Check sheet for the modelled part. Datum: model origin and axes. Units: mm. Give positions to 0.01 mm unless a question says otherwise; leave off trailing zeros. Write each loop counter-clockwise with the first axis right and the second up, starting at its lowest first coordinate (ties: lowest second). Pieces come first, ordered by that corner, then holes. Notation, with made-up numbers: (-16.5, 68.25) -> (20.5, 68.25) arc R27 cw to (20.5, 104.25) -> close; hole circle Ø8 at (-23, 48). An arc over 180 degrees is marked (long way). Use a Markdown table: item, result. Add a question column.
1. Cross-section at A-A (x = 96). Enter the section's corners in (y, z) (3 decimals).
2. Gauge pin test, flat ends, axial feed: P1, Ø10, axis at x = 73, y = 5.5, coming from the -Z side; P2, Ø4, axis at x = 53.5, z = -3.5, coming from the +Y side; P3, Ø4, axis at x = 69, y = -4.5, coming from the +Z side. Record the tip position at first contact, or that the pin passes through.
3. Scan lines: probe 1 along Y at (x, z) = (25, 6); probe 2 along Y at (x, z) = (99.5, 5.75); probe 3 along Z at (x, y) = (114, -4.75). Record each from-to range of solid material in increasing order. Write a range as [from, to].
from build123d import *

# Parameters (mm, degrees)
SKETCH1_W           = 120.675
SKETCH1_H           = 1.5875
CUT_EXTRUDE2_START  = 19.25
SKETCH4_R           = 12.7
CUT_EXTRUDE2_DEPTH  = 22.225
SKETCH6_R           = 7.9375
BOSS_EXTRUDE1_DEPTH = 101.6
SKETCH7_R           = 23.308025585
CUT_EXTRUDE3_DEPTH  = 19.075


with BuildPart() as part:
    # Sketch1 → Revolve1 (revolve)
    with BuildSketch(Plane(origin=(0, 0, 0), x_dir=(1, 0, 0), z_dir=(0, 1, 0))):
        with Locations((79.5875, 8.73125)):
            Rectangle(SKETCH1_W, SKETCH1_H)
    revolve(axis=Axis((157.324, 0, 0), (-1, 0, 0)))

    # Sketch4 → Cut-Extrude2 (cut)
    with BuildSketch(Plane(origin=(0, 0, 0), x_dir=(0, 0, -1), z_dir=(1, 0, 0)).offset(CUT_EXTRUDE2_START)):
        Circle(SKETCH4_R)
        Polygon((-9.235721046, 0.808020891), (-8.681700155, 0.254), (-8.681700155, -0.254), (-9.235721046, -0.808020891), (-8.593912259, -1.257420242), (-8.505698985, -1.75770258), (-8.955098336, -2.399511367), (-8.245002688, -2.730634406), (-8.071256455, -3.207998257), (-8.402379494, -3.918093905), (-7.645572882, -4.120879625), (-7.391572882, -4.56082053), (-7.594358603, -5.317627141), (-6.813836213, -5.385914002), (-6.487300108, -5.775064579), (-6.555586968, -6.555586968), (-5.775064579, -6.487300108), (-5.385914002, -6.813836213), (-5.317627141, -7.594358603), (-4.56082053, -7.391572882), (-4.120879625, -7.645572882), (-3.918093905, -8.402379494), (-3.207998257, -8.071256455), (-2.730634406, -8.245002688), (-2.399511367, -8.955098336), (-1.75770258, -8.505698985), (-1.257420242, -8.593912259), (-0.808020891, -9.235721046), (-0.254, -8.681700155), (0.254, -8.681700155), (0.808020891, -9.235721046), (1.257420242, -8.593912259), (1.75770258, -8.505698985), (2.399511367, -8.955098336), (2.730634406, -8.245002688), (3.207998257, -8.071256455), (3.918093905, -8.402379494), (4.120879625, -7.645572882), (4.56082053, -7.391572882), (5.317627141, -7.594358603), (5.385914002, -6.813836213), (5.775064579, -6.487300108), (6.555586968, -6.555586968), (6.487300108, -5.775064579), (6.813836213, -5.385914002), (7.594358603, -5.317627141), (7.391572882, -4.56082053), (7.645572882, -4.120879625), (8.402379494, -3.918093905), (8.071256455, -3.207998257), (8.245002688, -2.730634406), (8.955098336, -2.399511367), (8.505698985, -1.75770258), (8.593912259, -1.257420242), (9.235721046, -0.808020891), (8.681700155, -0.254), (8.681700155, 0.254), (9.235721046, 0.808020891), (8.593912259, 1.257420242), (8.505698985, 1.75770258), (8.955098336, 2.399511367), (8.245002688, 2.730634406), (8.071256455, 3.207998257), (8.402379494, 3.918093905), (7.645572882, 4.120879625), (7.391572882, 4.56082053), (7.594358603, 5.317627141), (6.813836213, 5.385914002), (6.487300108, 5.775064579), (6.555586968, 6.555586968), (5.775064579, 6.487300108), (5.385914002, 6.813836213), (5.317627141, 7.594358603), (4.56082053, 7.391572882), (4.120879625, 7.645572882), (3.918093905, 8.402379494), (3.207998257, 8.071256455), (2.730634406, 8.245002688), (2.399511367, 8.955098336), (1.75770258, 8.505698985), (1.257420242, 8.593912259), (0.808020891, 9.235721046), (0.254, 8.681700155), (-0.254, 8.681700155), (-0.808020891, 9.235721046), (-1.257420242, 8.593912259), (-1.75770258, 8.505698985), (-2.399511367, 8.955098336), (-2.730634406, 8.245002688), (-3.207998257, 8.071256455), (-3.918093905, 8.402379494), (-4.120879625, 7.645572882), (-4.56082053, 7.391572882), (-5.317627141, 7.594358603), (-5.385914002, 6.813836213), (-5.775064579, 6.487300108), (-6.555586968, 6.555586968), (-6.487300108, 5.775064579), (-6.813836213, 5.385914002), (-7.594358603, 5.317627141), (-7.391572882, 4.56082053), (-7.645572882, 4.120879625), (-8.402379494, 3.918093905), (-8.071256455, 3.207998257), (-8.245002688, 2.730634406), (-8.955098336, 2.399511367), (-8.505698985, 1.75770258), (-8.593912259, 1.257420242), align=None, mode=Mode.SUBTRACT)
    extrude(amount=CUT_EXTRUDE2_DEPTH, mode=Mode.SUBTRACT)

    # Sketch6 → Boss-Extrude1 (add)
    with BuildSketch(Plane.ZY.offset(-19.25)):
        Circle(SKETCH6_R)
    extrude(amount=-BOSS_EXTRUDE1_DEPTH)

    # Sketch7 → Cut-Extrude3 (cut)
    with BuildSketch(Plane(origin=(120.85, 0, 0), x_dir=(0, 0, -1), z_dir=(1, 0, 0))):
        Circle(SKETCH7_R)
    extrude(amount=CUT_EXTRUDE3_DEPTH, mode=Mode.SUBTRACT)


solid = part.part
Worked answers:
| question | item | result |
|---|---|---|
| 1 | outline | circle Ø19.05 at (0, 0) |
| 2 | P1 | stops at z = -9.51 |
| 2 | P2 | stops at y = 9.41 |
| 2 | P3 | stops at z = 9.19 |
| 3 | probe 1 | y = [-6.51, 6.51] |
| 3 | probe 2 | y = [-7.59, 7.59] |
| 3 | probe 3 | z = [-8.26, 8.26] |
